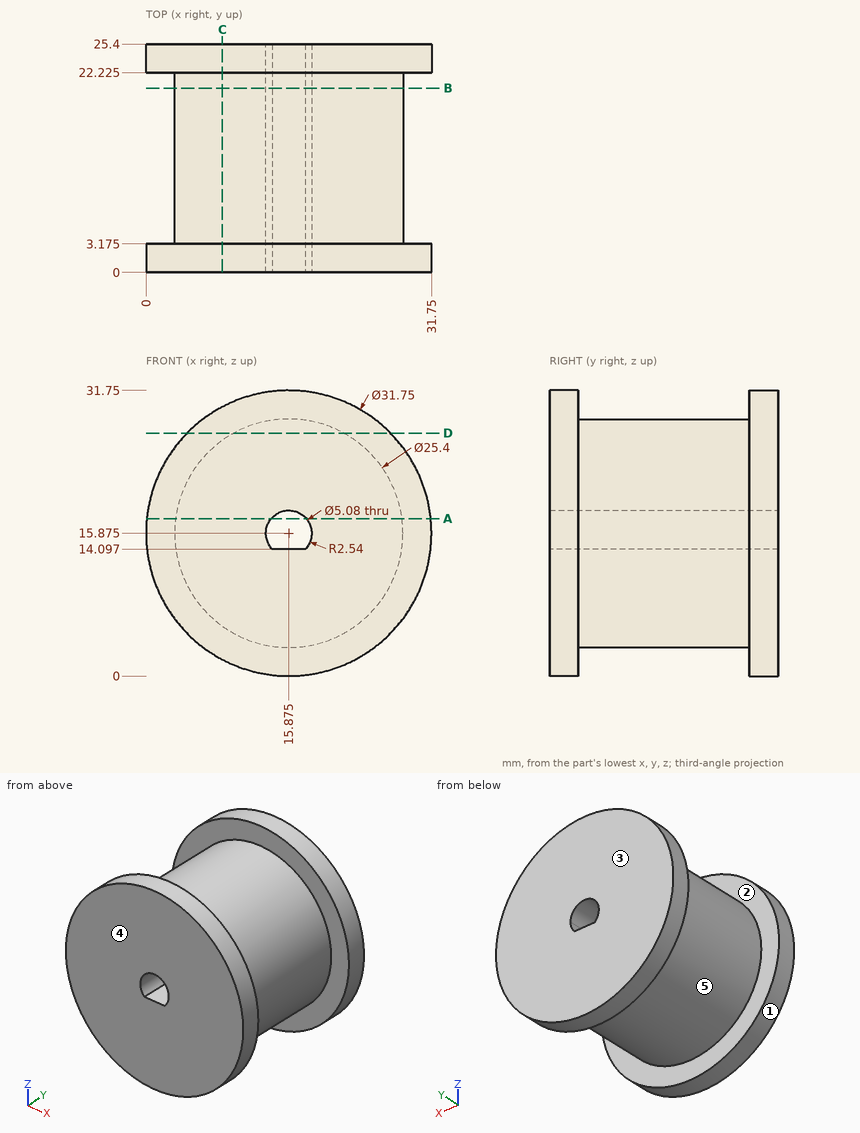
Geometry: see drawing. Coordinates: mm, zero at the bounding-box minimum. A direction names the side the tool comes from. Give positions to 0.01 mm unless a question says otherwise; leave off trailing zeros. Loops run counter-clockwise (first coordinate to the right, second up) from the corner with the lowest first, then second, coordinate; pieces in that order, holes last. Notation, with made-up numbers: (18.25, 35.5) - (67.25, 35.5) arc R9 ccw to (67.25, 50.5) - close; hole circle Ø3 at (39, -0.5). An arc over 180 degrees is marked (long way). Use CSV: the item, a comma, the result in double quotes. Start each with the question number.
1. Section C-C (x = 8.5). Output: boundary loops of the cut face in (y, z) (3 decimals).
2. Ray query, L1, parallel to Y at x = 9.5, z = 4 (3 decimals); L2, parallel to Z at x = 16, y = 2; L3, parallel to X at y = 16.75, z = 16.5. Return the intervals inside material, ascending.
3. Section D-D (z = 27). Output: boundary loops of the cut face in (x, y) (3 decimals).
4. Pin query (flat end, axial travel): pin 1 (6 mm diameter, centred on y = 7.5, z = 18.5, fed in from +X) (3 decimals); pin 2 (2 mm diameter, centred on x = 15.5, y = 9, fed in from +Z) (3 decimals); pin 3 (12 mm diameter, centred on y = 12, z = 21.5, fed in from -X) (3 decimals). Return the tip coordinate at first contact, or that it passes through.
5. Section B-B (y = 20.5). Output: boundary loops of the cut face in (x, z) (3 decimals).
6. Reachability of the marked faces 4 and 5 from +Z, -Z, +X, -X, +Y, -Y: full face, straight path, thin tool, end or side. Return the list, or none.
7. Section A-A (z = 17.5). Output: boundary loops of the cut face in (x, y) (3 decimals).
8. Draft query along Y for the marked faces 1, 2 and 3. Return one class per face: +Y half, -Y half, draft (parallel to the pull), parting line (faces both ways), or undercut.
Response:
1,outline,"(0, 1.817) - (3.175, 1.817) - (3.175, 5.536) - (22.225, 5.536) - (22.225, 1.817) - (25.4, 1.817) - (25.4, 29.933) - (22.225, 29.933) - (22.225, 26.214) - (3.175, 26.214) - (3.175, 29.933) - (0, 29.933) - close"
2,L1,"0 to 3.175, 22.225 to 25.4"
2,L2,"0 to 14.1, 18.41 to 31.75"
2,L3,"3.19 to 13.41, 18.34 to 28.56"
3,outline,"(4.55, 0) - (27.2, 0) - (27.2, 3.175) - (22.001, 3.175) - (22.001, 22.225) - (27.2, 22.225) - (27.2, 25.4) - (4.55, 25.4) - (4.55, 22.225) - (9.749, 22.225) - (9.749, 3.175) - (4.55, 3.175) - close"
4,pin 1,"x = 28.575"
4,pin 2,"z = 28.575"
4,pin 3,"x = 3.175"
5,outline,"circle Ø25.4 at (15.875, 15.875); hole (14.061, 14.097) - (17.689, 14.097) arc R2.54 ccw (long way) to start"
6,face 4,"+Z, -Z, +X, -X, -Y"
6,face 5,"none"
7,outline,"(0.083, 0) - (13.923, 0) - (13.923, 25.4) - (0.083, 25.4) - (0.083, 22.225) - (3.279, 22.225) - (3.279, 3.175) - (0.083, 3.175) - close; (17.827, 0) - (31.667, 0) - (31.667, 3.175) - (28.471, 3.175) - (28.471, 22.225) - (31.667, 22.225) - (31.667, 25.4) - (17.827, 25.4) - close"
8,face 1,"draft"
8,face 2,"undercut"
8,face 3,"+Y half"
